```python
from build123d import *

# Parameters (mm, degrees)
SKETCH1_R                        = 10.4521
SKETCH1_R_2                      = 4.9276
BASE_DEPTH                       = 1.1938
SKETCH2_R                        = 9.6393
SKETCH2_R_2                      = 8.89
TRACK_DEPTH                      = 0.7112
SKETCH3_R                        = 1.9431
PLATFORM_A1_DEPTH                = 0.3302
SKETCH4_R                        = 1.4859
PLATFORM_A2_DEPTH                = 3.175
SKETCH5_R                        = 0.9906
PLATFORM_A3_DEPTH                = 1.397
CCW_PATTERN_FOR_PLATFORM_A_COUNT = 2
CCW_PATTERN_FOR_PLATFORM_A_ANGLE = 115
CW_PATTERN_FOR_PLATFORM_A_COUNT  = 2
CW_PATTERN_FOR_PLATFORM_A_ANGLE  = 115
SKETCH6_R                        = 1.9431
PLATFORM_B1_DEPTH                = 0.3302
SKETCH7_R                        = 0.9779
PLATFORM_B2_DEPTH                = 3.175
SKETCH8_R                        = 0.7366
PLATFORM_B3_DEPTH                = 1.397
CCW_PATTERN_FOR_PLATFORM_B_COUNT = 2
CCW_PATTERN_FOR_PLATFORM_B_ANGLE = 113
CW_PATTERN_FOR_PLATFORM_B_COUNT  = 2
CW_PATTERN_FOR_PLATFORM_B_ANGLE  = 113


with BuildPart() as part:
    # Sketch1 → Base (new body)
    with BuildSketch(Plane.XY):
        Circle(SKETCH1_R)
        Circle(SKETCH1_R_2, mode=Mode.SUBTRACT)
    extrude(amount=BASE_DEPTH)

    # Sketch2 → Track (add)
    with BuildSketch(Plane(origin=(0, 0, 0), x_dir=(-1, 0, 0), z_dir=(0, 0, -1))):
        Circle(SKETCH2_R)
        Circle(SKETCH2_R_2, mode=Mode.SUBTRACT)
    extrude(amount=TRACK_DEPTH)

    # Sketch3 → Platform A1 (add)
    with BuildSketch(Plane.XY.offset(1.1938)):
        with Locations((0, 8.128)):
            Circle(SKETCH3_R)
    platform_a1 = extrude(amount=PLATFORM_A1_DEPTH)

    # Sketch4 → Platform A2 (add)
    with BuildSketch(Plane.XY.offset(1.524)):
        with Locations((0, 8.128)):
            Circle(SKETCH4_R)
    platform_a2 = extrude(amount=PLATFORM_A2_DEPTH)

    # Sketch5 → Platform A3 (add)
    with BuildSketch(Plane.XY.offset(4.699)):
        with Locations((0, 8.128)):
            Circle(SKETCH5_R)
    platform_a3 = extrude(amount=PLATFORM_A3_DEPTH)

    # CCW pattern for platform A: Platform A1, Platform A2, Platform A3 ×2 about axis
    ccw_pattern_for_platform_a_axis = Axis((0, 0, 1.1938), (0, 0, 1))
    for i in range(1, CCW_PATTERN_FOR_PLATFORM_A_COUNT):
        add(platform_a1.rotate(ccw_pattern_for_platform_a_axis, i * CCW_PATTERN_FOR_PLATFORM_A_ANGLE / (CCW_PATTERN_FOR_PLATFORM_A_COUNT - 1)))
        add(platform_a2.rotate(ccw_pattern_for_platform_a_axis, i * CCW_PATTERN_FOR_PLATFORM_A_ANGLE / (CCW_PATTERN_FOR_PLATFORM_A_COUNT - 1)))
        add(platform_a3.rotate(ccw_pattern_for_platform_a_axis, i * CCW_PATTERN_FOR_PLATFORM_A_ANGLE / (CCW_PATTERN_FOR_PLATFORM_A_COUNT - 1)))

    # CW pattern for platform A: Platform A1, Platform A2, Platform A3 ×2 about axis
    cw_pattern_for_platform_a_axis = Axis((0, 0, 1.1938), (0, 0, -1))
    for i in range(1, CW_PATTERN_FOR_PLATFORM_A_COUNT):
        add(platform_a1.rotate(cw_pattern_for_platform_a_axis, i * CW_PATTERN_FOR_PLATFORM_A_ANGLE / (CW_PATTERN_FOR_PLATFORM_A_COUNT - 1)))
        add(platform_a2.rotate(cw_pattern_for_platform_a_axis, i * CW_PATTERN_FOR_PLATFORM_A_ANGLE / (CW_PATTERN_FOR_PLATFORM_A_COUNT - 1)))
        add(platform_a3.rotate(cw_pattern_for_platform_a_axis, i * CW_PATTERN_FOR_PLATFORM_A_ANGLE / (CW_PATTERN_FOR_PLATFORM_A_COUNT - 1)))

    # Sketch6 → Platform B1 (add)
    with BuildSketch(Plane.XY.offset(1.1938)):
        with Locations((0, -8.0645)):
            Circle(SKETCH6_R)
    platform_b1 = extrude(amount=PLATFORM_B1_DEPTH)

    # Sketch7 → Platform B2 (add)
    with BuildSketch(Plane.XY.offset(1.524)):
        with Locations((0, -8.0645)):
            Circle(SKETCH7_R)
    platform_b2 = extrude(amount=PLATFORM_B2_DEPTH)

    # Sketch8 → Platform B3 (add)
    with BuildSketch(Plane.XY.offset(4.699)):
        with Locations((0, -8.0645)):
            Circle(SKETCH8_R)
    platform_b3 = extrude(amount=PLATFORM_B3_DEPTH)

    # CCW pattern for platform B: Platform B1, Platform B2, Platform B3 ×2 about axis
    ccw_pattern_for_platform_b_axis = Axis((0, 0, 1.1938), (0, 0, 1))
    for i in range(1, CCW_PATTERN_FOR_PLATFORM_B_COUNT):
        add(platform_b1.rotate(ccw_pattern_for_platform_b_axis, i * CCW_PATTERN_FOR_PLATFORM_B_ANGLE / (CCW_PATTERN_FOR_PLATFORM_B_COUNT - 1)))
        add(platform_b2.rotate(ccw_pattern_for_platform_b_axis, i * CCW_PATTERN_FOR_PLATFORM_B_ANGLE / (CCW_PATTERN_FOR_PLATFORM_B_COUNT - 1)))
        add(platform_b3.rotate(ccw_pattern_for_platform_b_axis, i * CCW_PATTERN_FOR_PLATFORM_B_ANGLE / (CCW_PATTERN_FOR_PLATFORM_B_COUNT - 1)))

    # CW pattern for platform B: Platform B1, Platform B2, Platform B3 ×2 about axis
    cw_pattern_for_platform_b_axis = Axis((0, 0, 1.1938), (0, 0, -1))
    for i in range(1, CW_PATTERN_FOR_PLATFORM_B_COUNT):
        add(platform_b1.rotate(cw_pattern_for_platform_b_axis, i * CW_PATTERN_FOR_PLATFORM_B_ANGLE / (CW_PATTERN_FOR_PLATFORM_B_COUNT - 1)))
        add(platform_b2.rotate(cw_pattern_for_platform_b_axis, i * CW_PATTERN_FOR_PLATFORM_B_ANGLE / (CW_PATTERN_FOR_PLATFORM_B_COUNT - 1)))
        add(platform_b3.rotate(cw_pattern_for_platform_b_axis, i * CW_PATTERN_FOR_PLATFORM_B_ANGLE / (CW_PATTERN_FOR_PLATFORM_B_COUNT - 1)))


solid = part.part
```
Check sheet for the modelled part. Datum: model origin and axes. Units: mm. A direction names the side the tool comes from. Round coordinates to 2 decimals unless told otherwise and drop trailing zeros. Loops run counter-clockwise (first coordinate to the right, second up) from the corner with the lowest first, then second, coordinate; pieces in that order, holes last. Notation, with made-up numbers: (-38, 22.25) - (18, 22.25) arc R25 ccw to (18, 59.25) - close; hole circle Ø3 at (31.5, -21). An arc over 180 degrees is marked (long way). Write item = value, one per line. Start each with the question number.
Q1. Section check B-B (z = 5). Record the boundary of the cut face in (x, y).
Q2. Depth check by flat-ended pin: P1, Ø3, axis at y = 0.5, z = 2.5, coming from the +X side; P2, Ø1, axis at x = 0, z = 3.5, coming from the +Y side; P3, Ø1.5, axis at x = 4, y = -5, coming from the -Z side; P4, Ø3, axis at y = 5.5, z = 2, coming from the +X side. Enter the tip coordinate at first touch or a pass-through.
Q3. Section check C-C (x = 2.25). Record the boundary of the cut face in (y, z).
Q4. Release check for a two-part mould opening along Y. For faces 1 (the face through (-7, -3, 6.096)), 2 (the face through (2.09, -9.41, -0.35)), 3 (the face through (1, -9, 1.524)) record: pulls with the +Y half, pulls with the -Y half, needs draft (parallel to the pull), parting line crosses it, or undercut.
Q5. Access from +Z, -Z, +X, -X, +Y, -Y to the whole of each face (thin tool, end or side, straight path). Record for faces 4 (the face through (7, -7, 0)), 5 (the face through (7.177, 2.457, 5.388)), 6 (the face through (-4.923, 0.217, 0.589)).
Q6. Thickness scan on L1, parallel to Y at x = 0, z = -0.2; L2, parallel to Y at x = 0, z = 4; L3, parallel to Z at x = 4.75, y = 3. Record the ranges inside material, lowest first.
Q7. Section check A-A (y = 0). Record the boundary of the cut face in (x, z).
Q8. Section check D-D (y = 5.5). Record the boundary of the cut face in (x, z), plus the area to 3 significant figures.
Derived:
q1.outline = circle Ø1.98 at (-7.37, -3.44); circle Ø1.47 at (-7.42, 3.15); circle Ø1.98 at (0, 8.13); circle Ø1.47 at (0, -8.06); circle Ø1.98 at (7.37, -3.44); circle Ø1.47 at (7.42, 3.15)
q2.P1 = 10.45
q2.P2 = 9.61
q2.P3 = 0
q2.P4 = 9.56
q3.outline = (-10.21, 0) - (-9.37, 0) - (-9.37, -0.71) - (-8.6, -0.71) - (-8.6, 0) - (-4.38, 0) - (-4.38, 1.19) - (-10.21, 1.19) - close; (4.38, 0) - (8.6, 0) - (8.6, -0.71) - (9.37, -0.71) - (9.37, 0) - (10.21, 0) - (10.21, 1.19) - (4.38, 1.19) - close
q4.face_1 = needs draft
q4.face_2 = parting line crosses it
q4.face_3 = undercut
q5.face_4 = -Z
q5.face_5 = +Z
q5.face_6 = +Z, -Z
q6.L1 = -9.64 to -8.89, 8.89 to 9.64
q6.L2 = -9.04 to -7.09, 6.64 to 9.61
q6.L3 = 0 to 1.19
q7.outline = (-10.45, 0) - (-9.64, 0) - (-9.64, -0.71) - (-8.89, -0.71) - (-8.89, 0) - (-4.93, 0) - (-4.93, 1.19) - (-10.45, 1.19) - close; (4.93, 0) - (8.89, 0) - (8.89, -0.71) - (9.64, -0.71) - (9.64, 0) - (10.45, 0) - (10.45, 1.19) - (4.93, 1.19) - close
q8.outline = (-8.89, 0) - (-7.92, 0) - (-7.92, -0.71) - (-6.98, -0.71) - (-6.98, 0) - (6.98, 0) - (6.98, -0.71) - (7.92, -0.71) - (7.92, 0) - (8.89, 0) - (8.89, 1.19) - (-8.89, 1.19) - close
q8.area = 22.5 mm^2
